from build123d import *

# Parameters (mm, degrees)
BOSS_EXTRUDE1_DEPTH   = 1.5
F_4_0MM_DOWEL_HOLE1_D = 3.5


with BuildPart() as part:
    # Sketch1 → Boss-Extrude1 (new body)
    with BuildSketch(Plane(origin=(0, 0, 0), x_dir=(1, 0, 0), z_dir=(0, 1, 0))):
        Polygon((0, 0), (-67.7, 0), (-67.7, -48.64), (-104.14, -48.64), (-104.14, -68.409681711), (-114.3, -68.409681711), (-114.300084457, -97.709681711), (-104.140084457, -97.709681711), (-104.140084457, -126.999681711), (-52.560084457, -126.999681711), (0, -67.34), align=None)
    extrude(amount=BOSS_EXTRUDE1_DEPTH)

    # Ø4.0mm Dowel Hole1 (through all)
    with Locations(Plane(origin=(-99.060084457, 1.5, 121.919681711), x_dir=(0, 0, 1), z_dir=(0, 1, 0))):
        with Locations((0, 0), (0, 43.21), (-58.839681711, 93.980084457), (-27.682634748, 68.593581655), (-116.839681711, 93.980084457), (-116.839681711, 36.440084457)):
            Hole(F_4_0MM_DOWEL_HOLE1_D / 2)


solid = part.part
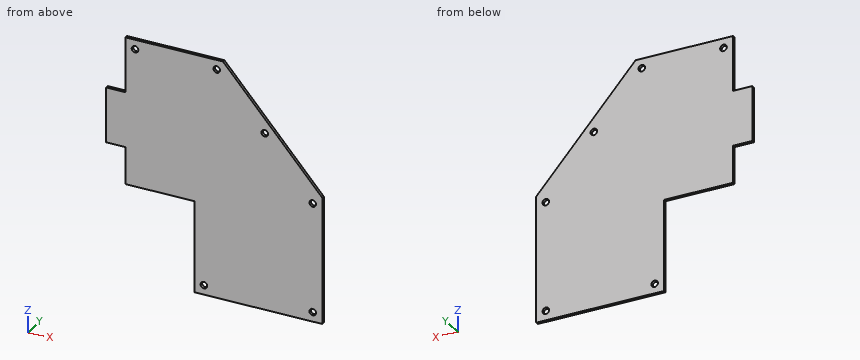
Geometry: final body of the model. Coordinates: model frame, mm. Give positions to 0.01 mm unless a question says otherwise; leave off trailing zeros. Write each loop counter-clockwise with the first axis right and the second up, starting at its lowest first coordinate (ties: lowest second). Pieces come first, ordered by that corner, then holes.
(1) Cut plane B-B, the plane x = -62.62. Return loops of the section in (y, z), then the cut area to 3 significant figures.
(2) Ray query, line 1 (X direction, y = 0.65, z = 5.08); line 2 (X direction, y = 0.9, z = 63.08); line 3 (Z direction, x = -62.62, y = 0.7). Return the intervals inside material, ascending.
(3) Cut plane D-D, the plane x = -5.08. Return loops of the section in (y, z).
(4) First-contact query: P1, Ø0.8, axis at y = 1, z = 16.5, coming from the -X side; P2, Ø3, axis at x = -99.06, z = 121.92, coming from the +Y side; P3, Ø0.8, axis at y = 1, z = 61, coming from the -X side; P4, Ø0.8, axis at x = -107, y = 1, coming from the +Z side. Flat tips, straight axial feed; report the tip coordinate or a pass-through.
(5) Cut plane C-C, the plane z = 5.08. Return loops of the section in (x, y).
(6) Cut plane A-A, the plane z = 63.08. Return loops of the section in (x, y), then the cut area to 3 significant figures.
Values follow:
1. outline: (0, 0) - (1.5, 0) - (1.5, 3.33) - (0, 3.33) - close; (0, 6.83) - (1.5, 6.83) - (1.5, 127) - (0, 127) - close
1. area: 185 mm2
2. line 1: x = -67.7 to -64.37, -60.87 to -6.83, -3.33 to 0
2. line 2: x = -104.14 to -6.83, -3.33 to 0
2. line 3: z = 0 to 3.33, 6.83 to 127
3. outline: (0, 0) - (1.5, 0) - (1.5, 3.33) - (0, 3.33) - close; (0, 6.83) - (1.5, 6.83) - (1.5, 61.33) - (0, 61.33) - close; (0, 64.83) - (1.5, 64.83) - (1.5, 73.11) - (0, 73.11) - close
4. P1: stops at x = -67.7
4. P2: passes through
4. P3: stops at x = -104.14
4. P4: stops at z = 97.71
5. outline: (-67.7, 0) - (-64.37, 0) - (-64.37, 1.5) - (-67.7, 1.5) - close; (-60.87, 0) - (-6.83, 0) - (-6.83, 1.5) - (-60.87, 1.5) - close; (-3.33, 0) - (0, 0) - (0, 1.5) - (-3.33, 1.5) - close
6. outline: (-104.14, 0) - (-6.83, 0) - (-6.83, 1.5) - (-104.14, 1.5) - close; (-3.33, 0) - (0, 0) - (0, 1.5) - (-3.33, 1.5) - close
6. area: 151 mm2
